Can you work these out from the drawing? Everything is in mm from the part's minimum corner. A direction names the side the tool comes from. Round coordinates to 2 decimals unless told otherwise and drop trailing zeros. Order: outer loops, then holes, each group sorted by start corner. A loop starts at its lowest first (then second) coordinate and runs counter-clockwise, first axis right, second up. Notation, with made-up numbers: (88, 35.25) - (108, 35.25) arc R13 cw to (108, 49.25) - close; hole circle Ø3 at (15.5, 29.5). An arc over 180 degrees is marked (long way). Answer as a JSON object with one key per item and string values.
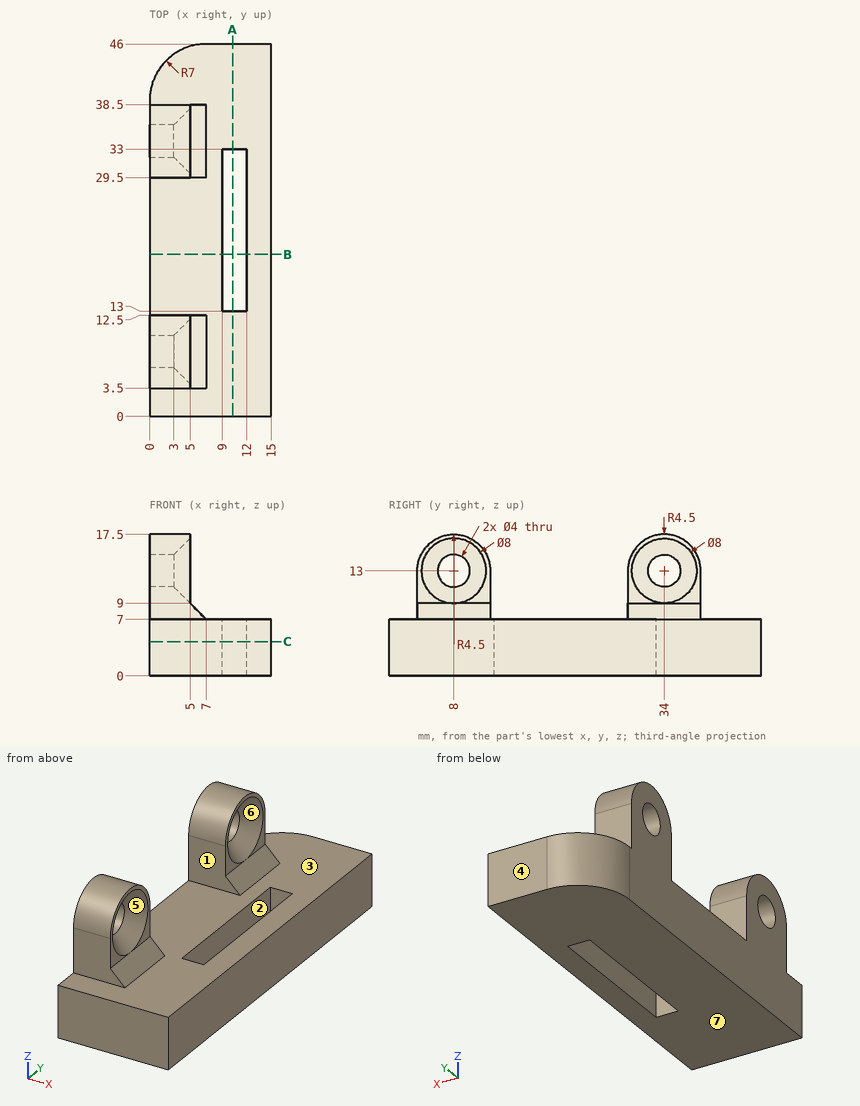
1. Imagine slicing it at B-B (y = 20). List the corners of the cut face in (x, z) for me.
Responses:
{"outline": "(0, 0) - (9, 0) - (9, 7) - (0, 7) - close; (12, 0) - (15, 0) - (15, 7) - (12, 7) - close"}
2. Imagine slicing it at C-C (z = 4.25). List the corners of the cut face in (x, y) for me.
Responses:
{"outline": "(0, 0) - (15, 0) - (15, 46) - (7, 46) arc R7 ccw to (0, 39) - close; hole (9, 13) - (12, 13) - (12, 33) - (9, 33) - close"}
3. For P1, Ø4.5, axis at x = 9, y = 22.5, coming from the +Z side; P2, Ø1.8, axis at x = 2, z = 11, coming from the +Y side; P3, Ø2, axis at x = 5, y = 39, coming from the +Z side, each with a flat end and sliding along its axis, tell me the tip position at first contact or that it passes through.
Responses:
{"P1": "z = 7", "P2": "y = 38.5", "P3": "z = 15.06"}
4. If I drill on L1, parallel to Z at x = 0.8, y = 34; L2, parallel to Y at x = 9.25, z = 2.75; L3, parallel to X at y = 13.5, z = 6.5, over which ranges is the centre line in solid material (lowest first)? Write a range as [from, to].
Responses:
{"L1": "[0, 11], [15, 17.5]", "L2": "[0, 13], [33, 46]", "L3": "[0, 9], [12, 15]"}
5. For the marked faces 1, 2 and 3, which set-ups out of +Z, -Z, +X, -X, +Y, -Y let a thin tool reach every point of the face, with its end or its side?
Responses:
{"face 1": "+Z, +X, -X", "face 2": "+Z, -Z", "face 3": "+Z, +X"}
6. Imagine slicing it at A-A (x = 10.25). List the corners of the cut face in (y, z) for me.
Responses:
{"outline": "(0, 0) - (13, 0) - (13, 7) - (0, 7) - close; (33, 0) - (46, 0) - (46, 7) - (33, 7) - close"}
7. Thinking about a two-plate mould opening in Z: for the marked faces 4, 5, 6 and 7, which applies, pulls with the +Z half, pulls with the -Z half, needs draft (parallel to the pull), parting line crosses it, or undercut?
Responses:
{"face 4": "needs draft", "face 5": "undercut", "face 6": "undercut", "face 7": "pulls with the -Z half"}
